from build123d import *

# Parameters (mm, degrees)
F0_W     = 137.6970596611
F0_H     = 76.2
F1_DEPTH = 10.922
F2_DEPTH = 25.4
F3_W     = 25.4
F3_H     = 5.08
F4_DEPTH = 25.4


with BuildPart() as f1:
    # F0 (on Front) → F1 (new body)
    with BuildSketch(Plane.XZ):
        with Locations((33.4425289184, 17.1839999914)):
            Rectangle(F0_W, F0_H)
    extrude(amount=F1_DEPTH)

    # F0 (on Front) → F2 (join)
    with BuildSketch(Plane.XZ):
        with Locations((33.4425289184, 17.1839999914)):
            Rectangle(F0_W, F0_H)
    extrude(amount=F2_DEPTH)

    # F3 (on face) → F4 (join)
    with BuildSketch(Plane.XY.offset(55.2839999914)):
        with Locations((33.1148739576, -10.16)):
            Rectangle(F3_W, F3_H)
    extrude(amount=F4_DEPTH)


solid = f1.part
Model file for the job. Use its own axes, mm. A direction names the side the tool comes from. Give positions to 0.01 mm unless a question says otherwise; leave off trailing zeros. Order: outer loops, then holes, each group sorted by start corner. A loop starts at its lowest first (then second) coordinate and runs counter-clockwise, first axis right, second up. Notation, with made-up numbers: M 4.5,8 L 40.5,8 A32 ccw 40.5,38 Z; hole C 69.5,35.25 d6. An arc over 180 degrees is marked long. Put each result on its own line as item: value. Start each with the question number.
(1) Drill centre lines: L1, parallel to Z at x = 63.5, y = -9; L2, parallel to X at y = -12.25, z = 68; L3, parallel to Y at x = 26, z = 55.5. Where is each one in solid material? Low to high. Write a range as [from, to].
(2) Band-saw the part on A-A on x = 35. Give the cut face in (y, z).
(3) Tool access for faces 1 (the face through (45.815, -10, 68)), 2 (the face through (33, -7.62, 68)), 3 (the face through (20.415, -10, 68)): list every direction of +Z, -Z, +X, -X, +Y, -Y with a clear straight run to the whole face (end or side of a thin tool).
(4) Pin check, flat tips, straight feed: pin 1 Ø12.5 at (x, z) = (38.5, 73) entering from +Y; pin 2 Ø10 at (x, y) = (0.5, -19) entering from +Z; pin 3 Ø1.5 at (y, z) = (-11.5, 70) entering from -X; pin 4 Ø10 at (x, z) = (78, 34.5) entering from +Y. Stop position of each tip, or through.
(5) Band-saw the part on C-C on z = 68. Give the cut face in (x, y).
(6) Band-saw the part on B-B on y = -23. Give the cut face in (x, z).
Results below:
1. L1: z = [-20.92, 55.28]
1. L2: x = [20.41, 45.81]
1. L3: y = [-12.7, -7.62]
2. outline: M -25.4,-20.92 L 0,-20.92 L 0,55.28 L -7.62,55.28 L -7.62,80.68 L -12.7,80.68 L -12.7,55.28 L -25.4,55.28 Z
3. face 1: +Z, +X, +Y, -Y
3. face 2: +Z, +X, -X, +Y
3. face 3: +Z, -X, +Y, -Y
4. pin 1: stops at y = -7.62
4. pin 2: stops at z = 55.28
4. pin 3: stops at x = 20.41
4. pin 4: stops at y = 0
5. outline: M 20.41,-12.7 L 45.81,-12.7 L 45.81,-7.62 L 20.41,-7.62 Z
6. outline: M -35.41,-20.92 L 102.29,-20.92 L 102.29,55.28 L -35.41,55.28 Z
